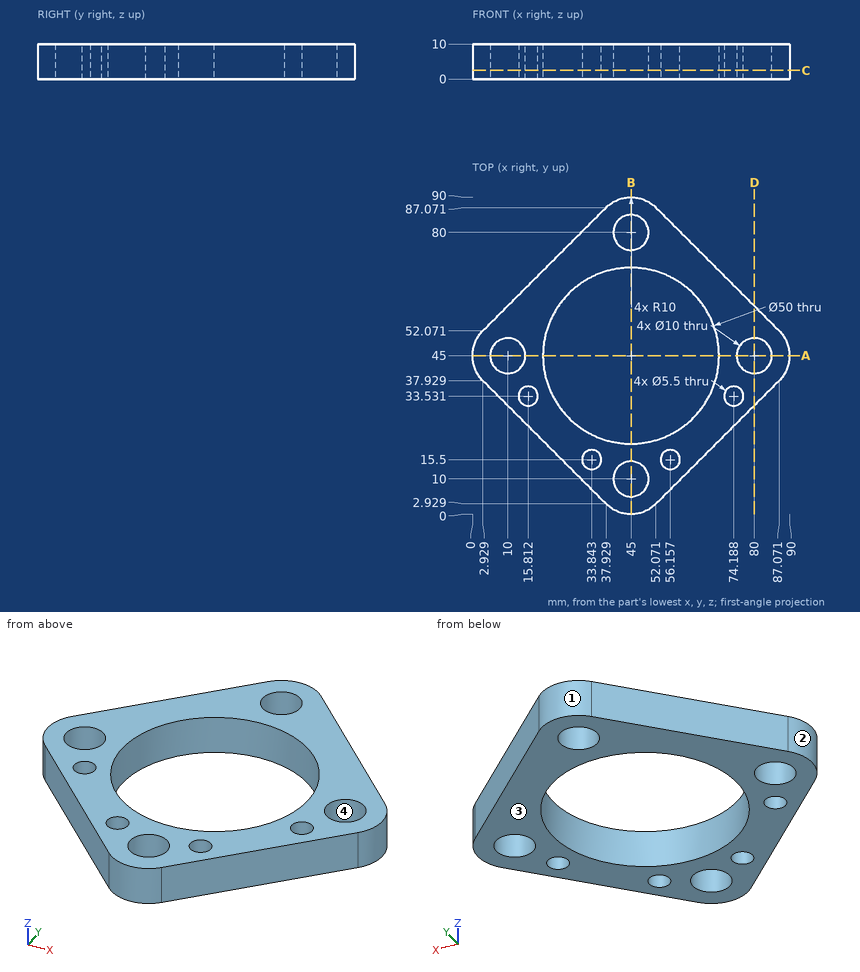
Study the drawing (mm; zero at the part's minimum x, y, z) and answer. Coordinates: 2 decimals unless noted, no trailing zeros. Write each loop counter-clockwise with the first axis right and the second up, starting at its lowest first coordinate (ties: lowest second). Pieces come first, ordered by that corner, then holes. Notation, with made-up numbers: (-25.5, 32) - (26.5, 32) arc R27 cw to (26.5, 70) - close; hole circle Ø5 at (-9, -8). An arc over 180 degrees is marked (long way). Return JSON: item names as keys, results as strings. Group by question number.
1. Straight lines are drawn through the part: L1, parallel to Y at x = 45, z = 5; L2, parallel to Y at x = 34.5, z = 3; L3, parallel to Y at x = 44, z = 9.25. For each, find the intervals that lie inside material, in ascending order.
2. Determine the mould class of the marked faces 1, 2, 3 and 4 for opening direction X: released by +X, released by -X, zero draft, split by the parting line, or undercut.
3. A cutting plane is placed at C-C, the plane z = 2.5. Give the number of separate pieces and of enclosed holes in the cut face, plus the area to 3 significant figures.
4. A cutting plane is placed at A-A, the plane y = 45. Determine the outline of the cut face in (x, z).
5. A cutting plane is placed at D-D, the plane x = 80. Determine the outline of the cut face in (y, z), plus the area to 3 significant figures.
6. Given pin 1 (3 mm diameter, centred on y = 34, z = 8.5, fed in from +X); pin 2 (2 mm diameter, centred on x = 22, z = 6.5, fed in from +Y); pin 3 (3 mm diameter, centred on x = 10.5, z = 1.5, fed in from -Y), each flat-ended and moving along its own axis, determine where each tip first touches the part or whether it passes through.
Ans:
{
 "1": {"L1": "0 to 5, 15 to 20, 70 to 75, 85 to 90", "L2": "6.36 to 12.83, 18.17 to 22.31, 67.69 to 83.64", "L3": "0.05 to 5.1, 14.9 to 20.02, 69.98 to 75.1, 84.9 to 89.95"},
 "2": {"face 1": "split by the parting line", "face 2": "released by -X", "face 3": "zero draft", "face 4": "undercut"},
 "3": {"separate pieces": "1", "enclosed holes": "9", "area": "2,370 mm²"},
 "4": {"outline": "(0, 0) - (5, 0) - (5, 10) - (0, 10) - close; (15, 0) - (20, 0) - (20, 10) - (15, 10) - close; (70, 0) - (75, 0) - (75, 10) - (70, 10) - close; (85, 0) - (90, 0) - (90, 10) - (85, 10) - close"},
 "5": {"outline": "(30.86, 0) - (40, 0) - (40, 10) - (30.86, 10) - close; (50, 0) - (59.14, 0) - (59.14, 10) - (50, 10) - close", "area": "183 mm²"},
 "6": {"pin 1": "x = 84.64", "pin 2": "y = 72.14", "pin 3": "y = 28.86"}
}
